For this review, take the finished solid that the model builds, in its own axes (mm). Face numbers are marked on the shaded views. A direction names the side the tool comes from. Coordinates: 2 decimals unless noted, no trailing zeros. Loops run counter-clockwise (first coordinate to the right, second up) from the corner with the lowest first, then second, coordinate; pieces in that order, holes last. Notation, with made-up numbers: (-15, 73.25) -> (-11, 73.25) arc R18 ccw to (-11, 93.25) -> close; hole circle Ø3 at (6.25, -14). An arc over 180 degrees is marked (long way). Answer in a Markdown table with one row per item.
from build123d import *

# Parameters (mm, degrees)
SKETCH3_R               = 3.075
CUT_EXTRUDE1_DEPTH      = 3.875
CUT_EXTRUDE1_DEPTH_BACK = 3.875


with BuildPart() as part:
    # Sketch1 → Revolve1 (revolve)
    with BuildSketch(Plane.XY):
        Polygon((-2.875, 1.5), (-2.875, 4.5), (-2.075, 4.5), (-2.075, 4), (2.075, 4), (2.075, 4.5), (2.875, 4.5), (2.875, 1.5), align=None)
    revolve(axis=Axis((0, 0, 0), (1, 0, 0)))

    # Sketch3 → Cut-Extrude1 (cut, two sides)
    with BuildSketch(Plane(origin=(0, 0, 0), x_dir=(0, 0, -1), z_dir=(1, 0, 0))) as cut_extrude1_sk:
        Circle(SKETCH3_R)
    extrude(amount=CUT_EXTRUDE1_DEPTH, mode=Mode.SUBTRACT)
    extrude(cut_extrude1_sk.sketch, amount=-CUT_EXTRUDE1_DEPTH_BACK, mode=Mode.SUBTRACT)


solid = part.part
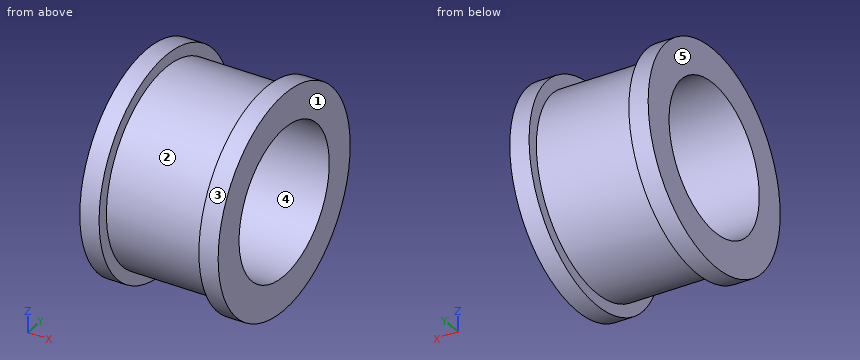
Item 1: Insertion check: pin 1 (1 mm diameter, centred on x = -2, y = 2, fed in from +Z); pin 2 (2.5 mm diameter, centred on y = -2, z = 0, fed in from -X) (3 decimals); pin 3 (1 mm diameter, centred on x = 1, z = -3, fed in from +Y); pin 4 (1 mm diameter, centred on x = 0.5, y = -3.5, fed in from +Z). Each pin has a flat end and moves straight along its axis. Give the tip position at first contact, or say it passes through.
Worked answers:
| item | result |
|---|---|
| pin 1 | z = 4.24 |
| pin 2 | x = -2.875 |
| pin 3 | y = 3.12 |
| pin 4 | z = 2.65 |
Item 2: For the marked faces 1 and 2, list the 3-axis set-ups (+Z, -Z, +X, -X, +Y, -Y) from which the entire face can be reached by the end or side of a thin tool; tool diameter is ignored.
Worked answers:
| item | result |
|---|---|
| face 1 | +Z, -Z, +X, +Y, -Y |
| face 2 | none |
Item 3: Take a section at D-D, the plane z = 3.25. State the section outline as (x, y) points (3 decimals).
Worked answers:
| item | result |
|---|---|
| outline | (-2.875, -3.112) -> (-2.075, -3.112) -> (-2.075, -2.332) -> (2.075, -2.332) -> (2.075, -3.112) -> (2.875, -3.112) -> (2.875, 3.112) -> (2.075, 3.112) -> (2.075, 2.332) -> (-2.075, 2.332) -> (-2.075, 3.112) -> (-2.875, 3.112) -> close |
Item 4: Take a section at C-C, the plane x = 1.35. State the section outline as (y, z) points (3 decimals).
Worked answers:
| item | result |
|---|---|
| outline | circle Ø8 at (0, 0); hole circle Ø6.15 at (0, 0) |
Item 5: The part is to be moulded in two halves that separate along Y. For the marked faces 3, 4 and 5, say which applies: +Y half, -Y half, draft (parallel to the pull), parting line (faces both ways), or undercut.
Worked answers:
| item | result |
|---|---|
| face 3 | parting line |
| face 4 | undercut |
| face 5 | draft |
Item 6: Take a section at A-A, the plane z = 0. State the section outline as (x, y) points (3 decimals), and give its area (3 significant figures).
Worked answers:
| item | result |
|---|---|
| outline | (-2.875, -4.5) -> (-2.075, -4.5) -> (-2.075, -4) -> (2.075, -4) -> (2.075, -4.5) -> (2.875, -4.5) -> (2.875, -3.075) -> (-2.875, -3.075) -> close; (-2.875, 3.075) -> (2.875, 3.075) -> (2.875, 4.5) -> (2.075, 4.5) -> (2.075, 4) -> (-2.075, 4) -> (-2.075, 4.5) -> (-2.875, 4.5) -> close |
| area | 12.2 mm² |
Item 7: For L1, parallel to Z at x = -1.7, y = 0 (3 decimals); L2, parallel to X at y = 4, z = 1 (3 decimals); L3, parallel to Z at x = -1.05, y = -2.5, list the stretches that pass through material, from the lowest coordinate up.
Worked answers:
| item | result |
|---|---|
| L1 | -4 to -3.075, 3.075 to 4 |
| L2 | -2.875 to -2.075, 2.075 to 2.875 |
| L3 | -3.12 to -1.79, 1.79 to 3.12 |
